Model file for the job. Use its own axes, mm. Face numbers are marked on the shaded views. A direction names the side the tool comes from. Coordinates: 2 decimals unless noted, no trailing zeros. Write each loop counter-clockwise with the first axis right and the second up, starting at its lowest first coordinate (ties: lowest second). Pieces come first, ordered by that corner, then holes. Notation, with made-up numbers: M -15.75,71 L 26.25,71 A14 ccw 26.25,82 Z; hole C -32.5,-9 d10. An arc over 180 degrees is marked long. Put each result on its own line as item: value. Start each with the question number.
Q1. Which spindle directions (+Z, -Z, +X, -X, +Y, -Y) get a long thin tool onto all of the face, cutting with end or side? Do the marked faces 1, 2 and 3. Say none if no direction does.
Q2. Cut at A-A (x = 0). Write the cut outline in (y, z), then the cut area to 3 significant figures.
Q3. Pull direction Y, two halves, no side cores. Call the marked faces 4, 5 and 6: pulls with the +Y half, pulls with the -Y half, needs draft (parallel to the pull), parting line crosses it, or undercut.
Q4. Drop flat-ended pins along their axis: pin 1 (2 mm diameter, centred on y = 4.5, z = 2.5, fed in from -X); pin 2 (3 mm diameter, centred on y = 11.5, z = -1.5, fed in from -X); pin 3 (3 mm diameter, centred on x = -2.5, y = 6.5, fed in from -Z). Give the stop position or say it passes through.
Q5. Cut at C-C (y = 20.5). Write the cut outline in (x, z), then the cut area to 3 significant figures.
Q6. Drill centre lines: line 1 along X through (y, z) = (14.5, -0.25); line 2 along Y through (x, z) = (3.75, 0.5); line 3 along Y through (x, z) = (3, -0.75). Where is each one in solid material? Low to high.
Q7. Cut at B-B (y = 25.5). Write the cut outline in (x, z), then the cut area to 3 significant figures.
```python
from build123d import *

# Parameters (mm, degrees)
BOSS_EXTRUDE1_DEPTH = 3
SKETCH2_R           = 2.35
BOSS_EXTRUDE2_DEPTH = 20
BOSS_EXTRUDE3_START = 23
BOSS_EXTRUDE3_DEPTH = 10
BOSS_EXTRUDE4_START = 30
SKETCH2_2_R         = 2.35
BOSS_EXTRUDE4_DEPTH = 4
CHAMFER1_SIZE       = 1.5


with BuildPart() as part:
    # Sketch1 → Boss-Extrude1 (new body)
    with BuildSketch(Plane(origin=(0, 0, 0), x_dir=(1, 0, 0), z_dir=(0, 1, 0))):
        Polygon((2.049593456, -3.55), (4.099186911, 0), (2.049593456, 3.55), (-2.049593456, 3.55), (-4.099186911, 0), (-2.049593456, -3.55), align=None)
    extrude(amount=BOSS_EXTRUDE1_DEPTH)

    # Sketch2 → Boss-Extrude2 (add)
    with BuildSketch(Plane(origin=(0, 3, 0), x_dir=(1, 0, 0), z_dir=(0, 1, 0))):
        with Locations(Location((0, 0, 0), (0, 0, 270))):
            Circle(SKETCH2_R)
    extrude(amount=BOSS_EXTRUDE2_DEPTH)

    # Sketch1<2> → Boss-Extrude3 (add)
    with BuildSketch(Plane(origin=(0, 0, 0), x_dir=(1, 0, 0), z_dir=(0, 1, 0)).offset(BOSS_EXTRUDE3_START)):
        Polygon((2.049593456, -3.55), (4.099186911, 0), (2.049593456, 3.55), (-2.049593456, 3.55), (-4.099186911, 0), (-2.049593456, -3.55), align=None)
    extrude(amount=BOSS_EXTRUDE3_DEPTH)

    # Sketch2<2> → Boss-Extrude4 (add)
    with BuildSketch(Plane(origin=(0, 3, 0), x_dir=(1, 0, 0), z_dir=(0, 1, 0)).offset(BOSS_EXTRUDE4_START)):
        with Locations(Location((0, 0, 0), (0, 0, 270))):
            Circle(SKETCH2_2_R)
    extrude(amount=BOSS_EXTRUDE4_DEPTH)

    # Chamfer1
    # the kernel refuses this chamfer: 1.5 mm, written as the material it adds along each edge
    with BuildSketch(Plane(origin=(0, 3, 0), x_dir=(0, 0, 1), z_dir=(-1, 0, 0))) as chamfer1_piece_1_section:
        Polygon((2.35, CHAMFER1_SIZE), (2.35 + CHAMFER1_SIZE, 0), (2.35, 0), align=None)
    chamfer1_piece_1 = revolve(axis=Axis((0, 3, 0), (0, 1, 0)), mode=Mode.PRIVATE)
    chamfer1_piece_1 = split(chamfer1_piece_1, bisect_by=Plane(origin=(4.408223306, 3.730355649, -0.535266737), z_dir=(-0.8660254037844387, 0, -0.5)), keep=Keep.TOP, mode=Mode.PRIVATE)
    chamfer1_piece_1 = split(chamfer1_piece_1, bisect_by=Plane(origin=(0, 3.730355649, 3.55), z_dir=(0, 0, -1)), keep=Keep.TOP, mode=Mode.PRIVATE)
    chamfer1_piece_1 = split(chamfer1_piece_1, bisect_by=Plane(origin=(1.740557061, 3.730355649, -4.085266737), z_dir=(-0.8660254037844387, 0, 0.5000000000000003)), keep=Keep.TOP, mode=Mode.PRIVATE)
    chamfer1_piece_1 = split(chamfer1_piece_1, bisect_by=Plane(origin=(-4.408223306, 3.730355649, -0.535266737), z_dir=(0.8660254037844387, 0, -0.5000000000000003)), keep=Keep.TOP, mode=Mode.PRIVATE)
    chamfer1_piece_1 = split(chamfer1_piece_1, bisect_by=Plane(origin=(0, 3.730355649, -3.55), z_dir=(0, 0, 1)), keep=Keep.TOP, mode=Mode.PRIVATE)
    chamfer1_piece_1 = split(chamfer1_piece_1, bisect_by=Plane(origin=(-1.740557061, 3.730355649, -4.085266737), z_dir=(0.8660254037844386, 0, 0.5000000000000002)), keep=Keep.TOP, mode=Mode.PRIVATE)
    add(chamfer1_piece_1)
    with BuildSketch(Plane(origin=(0, 23, 0), x_dir=(0, 0, 1), z_dir=(-1, 0, 0))) as chamfer1_piece_2_section:
        Polygon((2.35 + CHAMFER1_SIZE, 0), (2.35, -CHAMFER1_SIZE), (2.35, 0), align=None)
    chamfer1_piece_2 = revolve(axis=Axis((0, 23, 0), (0, 1, 0)), mode=Mode.PRIVATE)
    chamfer1_piece_2 = split(chamfer1_piece_2, bisect_by=Plane(origin=(4.408223304, 22.269644356, -0.535266733), z_dir=(-0.8660254037844387, 0, -0.5)), keep=Keep.TOP, mode=Mode.PRIVATE)
    chamfer1_piece_2 = split(chamfer1_piece_2, bisect_by=Plane(origin=(0, 22.269644356, 3.55), z_dir=(0, 0, -1)), keep=Keep.TOP, mode=Mode.PRIVATE)
    chamfer1_piece_2 = split(chamfer1_piece_2, bisect_by=Plane(origin=(1.740557063, 22.269644356, -4.085266733), z_dir=(-0.8660254037844387, 0, 0.5000000000000003)), keep=Keep.TOP, mode=Mode.PRIVATE)
    chamfer1_piece_2 = split(chamfer1_piece_2, bisect_by=Plane(origin=(-4.408223304, 22.269644356, -0.535266733), z_dir=(0.8660254037844387, 0, -0.5000000000000003)), keep=Keep.TOP, mode=Mode.PRIVATE)
    chamfer1_piece_2 = split(chamfer1_piece_2, bisect_by=Plane(origin=(0, 22.269644356, -3.55), z_dir=(0, 0, 1)), keep=Keep.TOP, mode=Mode.PRIVATE)
    chamfer1_piece_2 = split(chamfer1_piece_2, bisect_by=Plane(origin=(-1.740557063, 22.269644356, -4.085266733), z_dir=(0.8660254037844386, 0, 0.5000000000000002)), keep=Keep.TOP, mode=Mode.PRIVATE)
    add(chamfer1_piece_2)
    with BuildSketch(Plane(origin=(0, 33, 0), x_dir=(0, 0, 1), z_dir=(-1, 0, 0))) as chamfer1_piece_3_section:
        Polygon((2.35 + CHAMFER1_SIZE, 0), (2.35, CHAMFER1_SIZE), (2.35, 0), align=None)
    chamfer1_piece_3 = revolve(axis=Axis((0, 33, 0), (0, 1, 0)), mode=Mode.PRIVATE)
    chamfer1_piece_3 = split(chamfer1_piece_3, bisect_by=Plane(origin=(4.408223304, 33.730355644, -0.535266733), z_dir=(-0.8660254037844387, 0, -0.5)), keep=Keep.TOP, mode=Mode.PRIVATE)
    chamfer1_piece_3 = split(chamfer1_piece_3, bisect_by=Plane(origin=(0, 33.730355644, 3.55), z_dir=(0, 0, -1)), keep=Keep.TOP, mode=Mode.PRIVATE)
    chamfer1_piece_3 = split(chamfer1_piece_3, bisect_by=Plane(origin=(1.740557063, 33.730355644, -4.085266733), z_dir=(-0.8660254037844387, 0, 0.5000000000000003)), keep=Keep.TOP, mode=Mode.PRIVATE)
    chamfer1_piece_3 = split(chamfer1_piece_3, bisect_by=Plane(origin=(-4.408223304, 33.730355644, -0.535266733), z_dir=(0.8660254037844387, 0, -0.5000000000000003)), keep=Keep.TOP, mode=Mode.PRIVATE)
    chamfer1_piece_3 = split(chamfer1_piece_3, bisect_by=Plane(origin=(0, 33.730355644, -3.55), z_dir=(0, 0, 1)), keep=Keep.TOP, mode=Mode.PRIVATE)
    chamfer1_piece_3 = split(chamfer1_piece_3, bisect_by=Plane(origin=(-1.740557063, 33.730355644, -4.085266733), z_dir=(0.8660254037844386, 0, 0.5000000000000002)), keep=Keep.TOP, mode=Mode.PRIVATE)
    add(chamfer1_piece_3)


solid = part.part
```
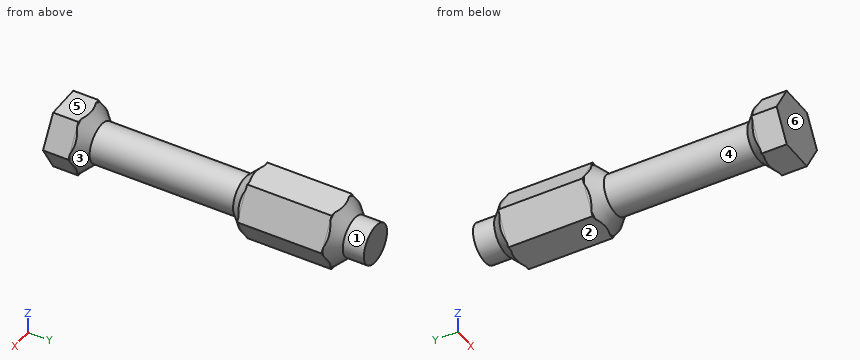
Computed values:
1. face 1: +Y
1. face 2: -Z, +X, -X, +Y, -Y
1. face 3: none
2. outline: M 0,-3.55 L 3.3,-3.55 L 4.5,-2.35 L 21.5,-2.35 L 22.7,-3.55 L 33.3,-3.55 L 34.5,-2.35 L 37,-2.35 L 37,2.35 L 34.5,2.35 L 33.3,3.55 L 22.7,3.55 L 21.5,2.35 L 4.5,2.35 L 3.3,3.55 L 0,3.55 Z
2. area: 212 mm2
3. face 4: undercut
3. face 5: needs draft
3. face 6: pulls with the -Y half
4. pin 1: x = -2.52
4. pin 2: x = -2.35
4. pin 3: z = -2.13
5. outline: C 0,0 d4.7
5. area: 17.3 mm2
6. line 1: -2.34 to 2.34
6. line 2: 0 to 3.07, 22.93 to 33.07
6. line 3: 0 to 3.76, 22.24 to 33.76
7. outline: M -4.1,0 L -2.05,-3.55 L 2.05,-3.55 L 4.1,0 L 2.05,3.55 L -2.05,3.55 Z
7. area: 43.7 mm2
